```python
from build123d import *

# Parameters (mm, degrees)
SKETCH1_W           = 76.2
SKETCH1_H           = 50.8
BOSS_EXTRUDE1_DEPTH = 7.62
SKETCH2_W           = 50.8
SKETCH2_H           = 13.97
CUT_EXTRUDE1_DEPTH  = 4.191
SKETCH3_W           = 8.89
SKETCH3_H           = 13.97
SKETCH3_W_2         = 19.685
CUT_EXTRUDE2_DEPTH  = 47.420193882
SKETCH4_R           = 2.38125
CUT_EXTRUDE3_DEPTH  = 47.420193882
SKETCH5_W           = 23.876
SKETCH5_H           = 3.3655
CUT_EXTRUDE4_DEPTH  = 47.420193882
SKETCH6_W           = 23.876
SKETCH6_H           = 1
CUT_EXTRUDE5_DEPTH  = 1.025400032
FILLET3_R           = 1.5875
FILLET6_R           = 1.5875
FILLET7_R           = 1.5875
SKETCH7_R           = 4.1275
CUT_EXTRUDE6_DEPTH  = 2.54


with BuildPart() as part:
    # Sketch1 → Boss-Extrude1 (new body)
    with BuildSketch(Plane(origin=(0, 0, 0), x_dir=(0, 1, 0), z_dir=(0, 0, 1))):
        Rectangle(SKETCH1_W, SKETCH1_H)
    extrude(amount=BOSS_EXTRUDE1_DEPTH)

    # Sketch2 → Cut-Extrude1 (cut)
    with BuildSketch(Plane.XY.offset(7.62)):
        Rectangle(SKETCH2_W, SKETCH2_H)
    extrude(amount=-CUT_EXTRUDE1_DEPTH, mode=Mode.SUBTRACT)

    # Sketch3 → Cut-Extrude2 (cut, through all)
    with BuildSketch(Plane(origin=(0, 0, 0), x_dir=(1, 0, 0), z_dir=(0, 0, -1))):
        with Locations((-20.955, 0)):
            Rectangle(SKETCH3_W, SKETCH3_H)
        with Locations((15.5575, 0)):
            Rectangle(SKETCH3_W_2, SKETCH3_H)
    extrude(amount=-CUT_EXTRUDE2_DEPTH, mode=Mode.SUBTRACT)

    # Sketch4 → Cut-Extrude3 (cut, through all)
    with BuildSketch(Plane.XY.offset(7.62)):
        with Locations((-17.78, 28.575)):
            Circle(SKETCH4_R)
        with Locations((-17.78, -28.575)):
            Circle(SKETCH4_R)
    extrude(amount=-CUT_EXTRUDE3_DEPTH, mode=Mode.SUBTRACT)

    # Sketch5 → Cut-Extrude4 (cut, through all)
    with BuildSketch(Plane.XY.offset(7.62)):
        with Locations((0, 28.575)):
            Rectangle(SKETCH5_W, SKETCH5_H)
        with Locations((0, -28.575)):
            Rectangle(SKETCH5_W, SKETCH5_H)
    extrude(amount=-CUT_EXTRUDE4_DEPTH, mode=Mode.SUBTRACT)

    # Sketch6 → Cut-Extrude5 (cut)
    with BuildSketch(Plane.XY.offset(7.62)):
        with Locations((0, 26.39225)):
            Rectangle(SKETCH6_W, SKETCH6_H)
        with Locations((0, -26.39225)):
            Rectangle(SKETCH6_W, SKETCH6_H)
        with Locations((0, 30.75775)):
            Rectangle(SKETCH6_W, SKETCH6_H)
        with Locations((0, -30.75775)):
            Rectangle(SKETCH6_W, SKETCH6_H)
    extrude(amount=-CUT_EXTRUDE5_DEPTH, mode=Mode.SUBTRACT)

    # Fillet3
    fillet3_edges = [part.edges().sort_by_distance(p)[0] for p in [
        (-16.51, 6.985, 1.7145),
        (-16.51, -6.985, 1.7145),
        (5.715, -6.985, 1.7145),
        (5.715, 6.985, 1.7145),
    ]]
    fillet(fillet3_edges, radius=FILLET3_R)

    # Fillet6
    fillet6_edges = [part.edges().sort_by_distance(p)[0] for p in [
        (-11.938, 30.25775, 3.297299984),
        (11.938, 30.25775, 3.297299984),
        (11.938, 26.89225, 3.297299984),
        (-11.938, 26.89225, 3.297299984),
        (-11.938, -26.89225, 3.297299984),
        (11.938, -26.89225, 3.297299984),
        (11.938, -30.25775, 3.297299984),
        (-11.938, -30.25775, 3.297299984),
    ]]
    fillet(fillet6_edges, radius=FILLET6_R)

    # Fillet7
    fillet7_edges = [part.edges().sort_by_distance(p)[0] for p in [
        (11.938, -31.25775, 7.107299984),
        (-11.938, -31.25775, 7.107299984),
        (-11.938, -25.89225, 7.107299984),
        (11.938, -25.89225, 7.107299984),
        (-11.938, 31.25775, 7.107299984),
        (11.938, 31.25775, 7.107299984),
        (11.938, 25.89225, 7.107299984),
        (-11.938, 25.89225, 7.107299984),
    ]]
    fillet(fillet7_edges, radius=FILLET7_R)

    # Sketch7 → Cut-Extrude6 (cut)
    with BuildSketch(Plane.XY.offset(7.62)):
        with Locations((-17.78, -28.575)):
            Circle(SKETCH7_R)
        with Locations((-17.78, 28.575)):
            Circle(SKETCH7_R)
    extrude(amount=-CUT_EXTRUDE6_DEPTH, mode=Mode.SUBTRACT)


solid = part.part
```
Could you check a few things on this model? Use its own coordinates, in mm. A direction names the side the tool comes from. Coordinates: 2 decimals unless noted, no trailing zeros. Write each loop counter-clockwise with the first axis right and the second up, starting at its lowest first coordinate (ties: lowest second). Pieces come first, ordered by that corner, then holes. Notation, with made-up numbers: (42, 89) - (99, 89) arc R26 ccw to (99, 127) - close; hole circle Ø10 at (-37, 60). An arc over 180 degrees is marked (long way). Use a Markdown table: item, result.
Q1. Imagine slicing it at D-D (y = 0.5). List the corners of the cut face in (x, z) for me (3 decimals), and give its area (3 significant figures).
Geometry check:
| item | result |
|---|---|
| outline | (-16.51, 0) - (5.715, 0) - (5.715, 3.429) - (-16.51, 3.429) - close |
| area | 76.2 mm2 |
Q2. Imagine slicing it at C-C (z = 1.75). Count the separate pieces of the cut face and the enclosed holes in it, and give its area (3 significant figures).
Geometry check:
| item | result |
|---|---|
| separate pieces | 1 |
| enclosed holes | 4 |
| area | 3,280 mm2 |
Q3. Imagine slicing it at A-A (x = -8.5). List the corners of the cut face in (y, z) for me (3 decimals), and give its area (3 significant figures).
Geometry check:
| item | result |
|---|---|
| outline | (-38.1, 0) - (-30.258, 0) - (-30.258, 6.595) - (-31.258, 6.595) - (-31.258, 7.62) - (-38.1, 7.62) - close; (-26.892, 0) - (26.892, 0) - (26.892, 6.595) - (25.892, 6.595) - (25.892, 7.62) - (6.985, 7.62) - (6.985, 3.429) - (-6.985, 3.429) - (-6.985, 7.62) - (-25.892, 7.62) - (-25.892, 6.595) - (-26.892, 6.595) - close; (30.258, 0) - (38.1, 0) - (38.1, 7.62) - (31.258, 7.62) - (31.258, 6.595) - (30.258, 6.595) - close |
| area | 467 mm2 |
Q4. I'm going to push flat-ended pins straight in: pin 1 Ø7 at (x, y) = (-2.5, 0.5) entering from +Z; pin 2 Ø1 at (y, z) = (-2.5, 1.5) entering from +X (3 decimals); pin 3 Ø3 at (x, y) = (-17.78, 28.575) entering from -Z; pin 4 Ø7.5 at (x, y) = (-17.78, 28.575) entering from +Z. Where does each tip first touch, or does it pass through?
Geometry check:
| item | result |
|---|---|
| pin 1 | stops at z = 3.43 |
| pin 2 | stops at x = 5.715 |
| pin 3 | passes through |
| pin 4 | stops at z = 5.08 |
Q5. Imagine slicing it at B-B (x = 20.5). List the corners of the cut face in (y, z) for me (3 decimals).
Geometry check:
| item | result |
|---|---|
| outline | (-38.1, 0) - (-6.985, 0) - (-6.985, 7.62) - (-38.1, 7.62) - close; (6.985, 0) - (38.1, 0) - (38.1, 7.62) - (6.985, 7.62) - close |
Q6. Thinking about a two-plate mould opening in X: for faces 1 (the flat face through (-16.51, 0, 2)), 2 (the flat face through (25.4, -23, 4)), 3 (the flat face through (0, -31, 6.595)), 4 (the cylindrical face through (-15.51, 29.29, 2.58)), which applies, +X half, -X half, draft (parallel to the pull), parting line (faces both ways), or undercut?
Geometry check:
| item | result |
|---|---|
| face 1 | -X half |
| face 2 | +X half |
| face 3 | undercut |
| face 4 | undercut |
Q7. Which directions (+Z, -Z, +X, -X, +Y, -Y) give clear straight access to the entire face, cutting with the end or side of a thin tool? Please do faces 5 (the cylindrical face through (11.485, 29.78, 3.251)), 6 (the flat face through (-25.4, 22, 4)), 7 (the cylindrical face through (-16.987, -6.532, 1.739)), 8 (the cylindrical face through (11.461, 30.805, 7.1)).
Geometry check:
| item | result |
|---|---|
| face 5 | +Z, -Z |
| face 6 | +Z, -Z, -X, +Y, -Y |
| face 7 | +Z, -Z, -X |
| face 8 | +Z |
Q8. Please list where these lines run through material, in increasing order: L1, parallel to Y at x = -17.78, z = 4.05 (3 decimals); L2, parallel to Y at x = -3, z = 5.5 (3 decimals); L3, parallel to Y at x = 1, z = 1.
Geometry check:
| item | result |
|---|---|
| L1 | y = -38.1 to -30.956, -26.194 to -6.985, 6.985 to 26.194, 30.956 to 38.1 |
| L2 | y = -38.1 to -30.258, -26.892 to -6.985, 6.985 to 26.892, 30.258 to 38.1 |
| L3 | y = -38.1 to -30.26, -26.89 to 26.89, 30.26 to 38.1 |
